Can you work these out from the model? Positions are in its coordinate system, mm. A direction names the side the tool comes from. Give positions to 0.01 mm unless a question says otherwise; leave off trailing zeros. Loops run counter-clockwise (first coordinate to the right, second up) from the corner with the lowest first, then second, coordinate; pieces in that order, holes last. Notation, with made-up numbers: (-13.5, -26) - (21.5, -26) arc R18 cw to (21.5, -5) - close; hole circle Ø6 at (-8.75, -17.5). An arc over 180 degrees is marked (long way). Answer in a Markdown table with one row per item.
Autodesk Inventor part; units mm, degrees
ref_plane "YZ Plane" through (0, 0, 0) normal (1, 0, 0) x (0, 1, 0)
ref_plane "XZ Plane" through (0, 0, 0) normal (0, 1, 0) x (-1, 0, 0)
ref_plane "XY Plane" through (0, 0, 0) normal (0, 0, 1) x (1, 0, 0)
sketch "Sketch1" plane through (0, 0, 0) normal (0, 0, 1) x (1, 0, 0)
  line L0 (-10.9985, 0) -> (-5.4993, 9.525)
  line L1 (-5.4993, 9.525) -> (5.4993, 9.525)
  line L2 (5.4993, 9.525) -> (10.9985, 0)
  line L3 (10.9985, 0) -> (5.4993, -9.525)
  line L4 (5.4993, -9.525) -> (-5.4993, -9.525)
  line L5 (-5.4993, -9.525) -> (-10.9985, 0)
  point P0 (0, 0)
  point P1 (0, 0)
  dimension "d0" = 19.05
extrude "Extrusion1" add sketch "Sketch1" against normal blind 3.81
sketch "Sketch2" plane through (0, 0, 0) normal (0, 0, 1) x (1, 0, 0)
  circle A0 centre (0, 0) radius 6.35
  dimension "d3" = 12.7
extrude "Extrusion2" add sketch "Sketch2" along normal blind 57.15
thread "Thread1"
properties part number "LucasCharles Part6 bolt for arm to speaker holder Final" material "Stainless Steel, Austenitic"
Q1. Imagine slicing it at B-B, the plane y = -3.5. Write out the boundary of the cut face in (x, z), and give its area (3 significant figures).
Checked values:
| item | result |
|---|---|
| outline | (-8.98, -3.81) - (8.98, -3.81) - (8.98, 0) - (5.3, 0) - (5.3, 57.15) - (-5.3, 57.15) - (-5.3, 0) - (-8.98, 0) - close |
| area | 674 mm² |
Q2. For pin 1 (3 mm diameter, centred on y = -1, z = 18.5, fed in from -X); pin 2 (2 mm diameter, centred on x = -1.5, z = 20.5, fed in from -Y); pin 3 (2 mm diameter, centred on x = -0.5, z = 27.5, fed in from +Y), each with a flat end and sliding along its axis, tell me the tip position at first contact or that it passes through.
Checked values:
| item | result |
|---|---|
| pin 1 | stops at x = -6.35 |
| pin 2 | stops at y = -6.33 |
| pin 3 | stops at y = 6.35 |
Q3. Imagine slicing it at D-D, the plane x = 8. Write out the boundary of the cut face in (y, z), and give its area (3 significant figures).
Checked values:
| item | result |
|---|---|
| outline | (-5.19, -3.81) - (5.19, -3.81) - (5.19, 0) - (-5.19, 0) - close |
| area | 39.6 mm² |
Q4. If I drill on line 1 (Z direction, x = 6, y = -5.5); line 2 (Y direction, x = 0, z = 18.5); line 3 (Y direction, x = 4.5, z = 14), over which ranges is the centre line in solid material (lowest first)? Write a range as [from, to].
Checked values:
| item | result |
|---|---|
| line 1 | z = [-3.81, 0] |
| line 2 | y = [-6.35, 6.35] |
| line 3 | y = [-4.48, 4.48] |
Q5. Imagine slicing it at C-C, the plane z = 52.5. Write out the boundary of the cut face in (x, y), and give its area (3 significant figures).
Checked values:
| item | result |
|---|---|
| outline | circle Ø12.7 at (0, 0) |
| area | 127 mm² |
Q6. Imagine slicing it at A-A, the plane x = 0. Write out the boundary of the cut face in (y, z) (3 decimals), and give its area (3 significant figures).
Checked values:
| item | result |
|---|---|
| outline | (-9.525, -3.81) - (9.525, -3.81) - (9.525, 0) - (6.35, 0) - (6.35, 57.15) - (-6.35, 57.15) - (-6.35, 0) - (-9.525, 0) - close |
| area | 798 mm² |
Q7. On a 3-axis mill with a long thin cutter (end or side, diameter ignored), from which of +Z, -Z, +X, -X, +Y, -Y can I reach the whole of each face in a straight line? I mean faces 1 (the face through (0, 0, 57.15)), 2 (the face through (-1.38, 6.2, 28.17)). Say none if no direction works.
Checked values:
| item | result |
|---|---|
| face 1 | +Z, +X, -X, +Y, -Y |
| face 2 | +Z |
